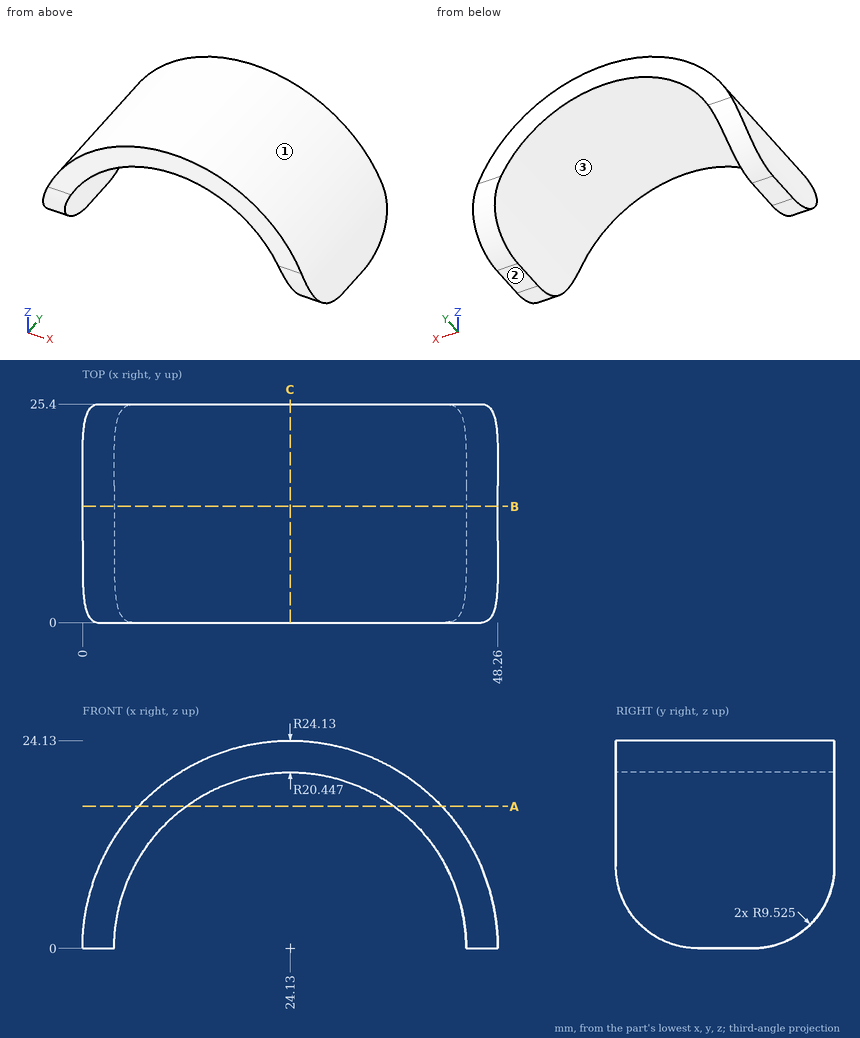
Can you work these out from the drawing? Everything is in mm from the part's minimum corner. Give positions to 0.01 mm unless a question says otherwise; leave off trailing zeros. Loops run counter-clockwise (first coordinate to the right, second up) from the corner with the lowest first, then second, coordinate; pieces in that order, holes last. Notation, with made-up numbers: (63, 42.5) -> (91, 42.5) arc R18 ccw to (91, 76.5) -> close; hole circle Ø5 at (51.5, 63). An arc over 180 degrees is marked (long way). Return JSON: item names as keys, results as strings.
Q1. For pin 1 Ø12 at (y, z) = (5.5, 16) entering from +X; pin 2 Ø12 at (x, y) = (41.5, 15.5) entering from +Z; pin 3 Ø3 at (y, z) = (4, 15) entering from +X, each with a flat end and sliding along its axis, tell me the tip position at first contact or that it passes through.
Checks:
{"pin 1": "stops at x = 46.09", "pin 2": "stops at z = 21.28", "pin 3": "stops at x = 44.13"}
Q2. I want a section at C-C, the plane x = 24.13. List the corners of the cut face in (y, z) for me, then the cut area to 3 significant figures.
Checks:
{"outline": "(0, 20.45) -> (25.4, 20.45) -> (25.4, 24.13) -> (0, 24.13) -> close", "area": "93.5 mm2"}
Q3. I need wall thicknesses on probe 1 along X at (y, z) = (4.75, 7.5); probe 2 along X at (y, z) = (13.25, 7.75); probe 3 along Y at (x, z) = (46, 5.5). Which ranges of each line are inside material? Lowest first, please.
Checks:
{"probe 1": "x = 1.2 to 5.11, 43.15 to 47.06", "probe 2": "x = 1.28 to 5.21, 43.05 to 46.98", "probe 3": "y = 0.89 to 24.51"}
Q4. I want a section at B-B, the plane y = 13.5. List the corners of the cut face in (x, z) for me.
Checks:
{"outline": "(0, 0) -> (3.68, 0) arc R20.45 cw to (44.58, 0) -> (48.26, 0) arc R24.13 ccw to start"}
Q5. I want a section at A-A, the plane z = 16.5. List the corners of the cut face in (x, y) for me, then the cut area to 3 significant figures.
Checks:
{"outline": "(6.52, 0) -> (12.05, 0) -> (12.05, 25.4) -> (6.52, 25.4) -> close; (36.21, 0) -> (41.74, 0) -> (41.74, 25.4) -> (36.21, 25.4) -> close", "area": "281 mm2"}
Q6. We'd pull the mould along X, two halves only. Please class the marked faces 1, 2 and 3: released by +X, released by -X, zero draft, split by the parting line, or undercut.
Checks:
{"face 1": "split by the parting line", "face 2": "zero draft", "face 3": "undercut"}
